Source: three-view drawing plus pictorial views. Frame: mm from the lowest corner of the part. A direction names the side the tool comes from. Coordinates: 2 decimals unless noted, no trailing zeros. Write each loop counter-clockwise with the first axis right and the second up, starting at its lowest first coordinate (ties: lowest second). Pieces come first, ordered by that corner, then holes. Notation, with made-up numbers: (21, 51.5) -> (80, 51.5) arc R38 cw to (80, 90.5) -> close; hole circle Ø6 at (-11, -34.75). An arc over 180 degrees is marked (long way). Write item = value, one per line.
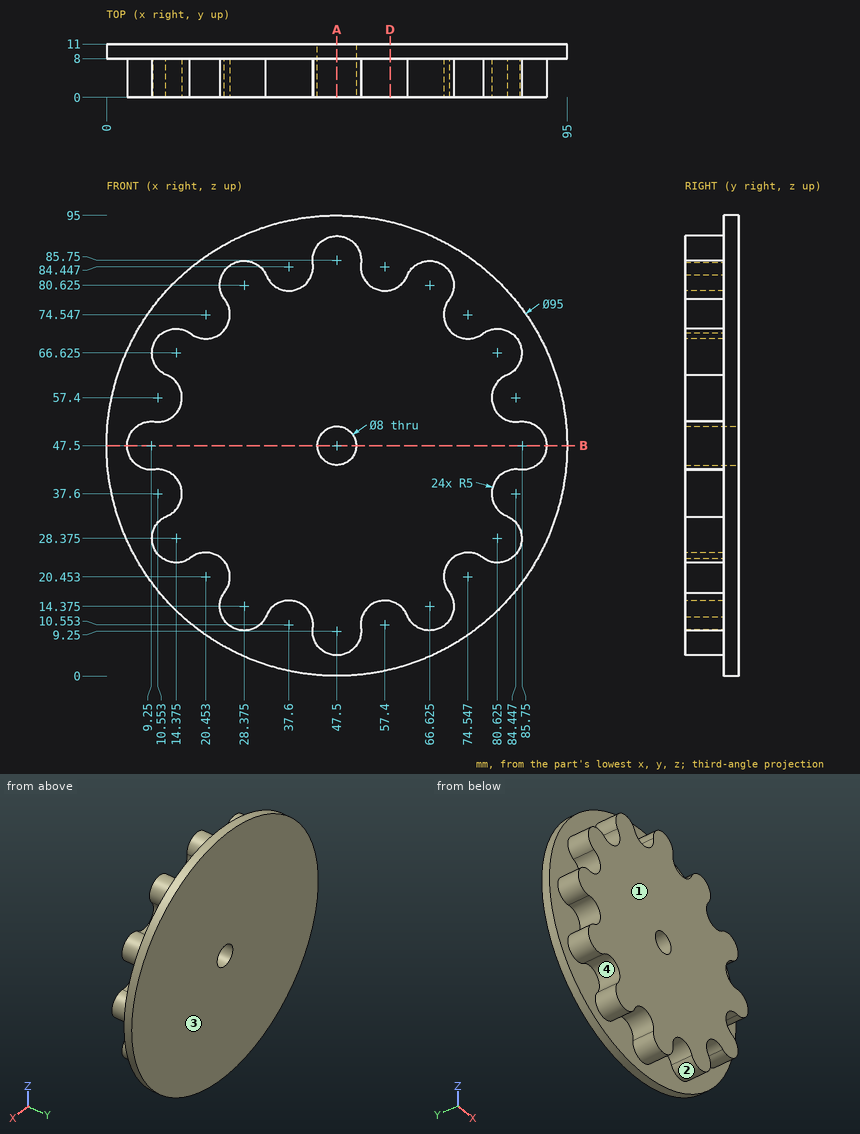
1) Reachability of the marked faces 3 and 4 from +Z, -Z, +X, -X, +Y, -Y: full face, straight path, thin tool, end or side. Return the list, or none.
Answer block:
face_3 = +Z, -Z, +X, -X, +Y
face_4 = -Y
2) Cut plane D-D, the plane x = 58.5. Output: boundary loops of the cut face in (y, z).
Answer block:
outline = (0, 15.43) -> (8, 15.43) -> (8, 1.29) -> (11, 1.29) -> (11, 93.71) -> (8, 93.71) -> (8, 79.57) -> (0, 79.57) -> close
3) Cut plane B-B, the plane z = 47.5. Output: boundary loops of the cut face in (x, y).
Answer block:
outline = (0, 8) -> (4.25, 8) -> (4.25, 0) -> (43.5, 0) -> (43.5, 11) -> (0, 11) -> close; (51.5, 0) -> (90.75, 0) -> (90.75, 8) -> (95, 8) -> (95, 11) -> (51.5, 11) -> close
4) First-contact query: pin 1 Ø4 at (x, y) = (26, 1.5) entering from -Z; pin 2 Ø3 at (x, y) = (50.5, 8) entering from -Z; pin 3 Ø9 at (x, z) = (47.5, 47.5) entering from -Y; pin 4 Ø1.5 at (y, z) = (2, 20.5) entering from +X. Flat tips, straight axial feed; report the tip coordinate or a pass-through.
Answer block:
pin_1 = 9.39
pin_2 = 0.02
pin_3 = 0
pin_4 = 69.61
5) Material intervals for probe 1 along X at (y, z) = (1.25, 11.5) (1 decimal); probe 2 along Z at (x, y) = (84, 6.5) (1 decimal); probe 3 along X at (y, z) = (6, 82), sorted ascending. Write a range as [from, to].
Answer block:
probe_1 = [24.3, 32.5], [42.5, 52.5], [62.5, 70.7]
probe_2 = [24.7, 32.1], [42.6, 52.4], [62.9, 70.3]
probe_3 = [23.57, 33.24], [41.96, 53.04], [61.76, 71.43]
6) Cut plane A-A, the plane x = 47.5. Output: boundary loops of the cut face in (y, z), and give its area (3 significant figures).
Answer block:
outline = (0, 4.25) -> (8, 4.25) -> (8, 0) -> (11, 0) -> (11, 43.5) -> (0, 43.5) -> close; (0, 51.5) -> (11, 51.5) -> (11, 95) -> (8, 95) -> (8, 90.75) -> (0, 90.75) -> close
area = 889 mm2
7) Pull-direction query (X, two-part tool) for the marked faces 1 and 2; classes: +X half, -X half, draft (parallel to the pull), parting line (faces both ways), or undercut.
Answer block:
face_1 = draft
face_2 = undercut
